```python
from build123d import *

# Parameters (mm, degrees)
SKETCH_1_R          = 2.1
SKETCH_1_R_2        = 1.599999998
SKETCH_1_R_3        = 2.099999998
SKETCH_1_R_4        = 1.6
EXTRUDE_1_DEPTH     = 3
FILLET_1_R          = 2
CUT_EXTRUDE_1_DEPTH = 115.739923305
SKETCH_3_W          = 8.5
SKETCH_3_H          = 7
CUT_EXTRUDE_2_DEPTH = 115.739923305
FILLET_2_R          = 3


with BuildPart() as part:
    # 草图1 → 凸台-拉伸1 (new body)
    with BuildSketch(Plane.XY):
        Polygon((-26, 0), (-26, -62), (26, -62), (26, -51), (96.5, -51), (96.5, -11), (26, -11), (26, 0), align=None)
        with Locations((-20, -4)):
            Circle(SKETCH_1_R, mode=Mode.SUBTRACT)
        with Locations((20, -4)):
            Circle(SKETCH_1_R, mode=Mode.SUBTRACT)
        with Locations((-20, -58)):
            Circle(SKETCH_1_R, mode=Mode.SUBTRACT)
        with Locations((20, -58)):
            Circle(SKETCH_1_R, mode=Mode.SUBTRACT)
        with Locations((42.500000002, -21.5)):
            Circle(SKETCH_1_R_2, mode=Mode.SUBTRACT)
        with Locations((42.500000002, -40.5)):
            Circle(SKETCH_1_R_2, mode=Mode.SUBTRACT)
        with Locations((92.500000002, -18)):
            Circle(SKETCH_1_R_3, mode=Mode.SUBTRACT)
        with Locations((92.500000002, -44)):
            Circle(SKETCH_1_R_3, mode=Mode.SUBTRACT)
        with Locations((25.75, -46)):
            Circle(SKETCH_1_R_4, mode=Mode.SUBTRACT)
        with Locations((25.75, -16)):
            Circle(SKETCH_1_R_4, mode=Mode.SUBTRACT)
        Polygon((68, -34.5), (68, -27.5), (40, -27.5), (40, -19), (24, -19), (24, -43), (40, -43), (40, -34.5), align=None, mode=Mode.SUBTRACT)
    extrude(amount=EXTRUDE_1_DEPTH)

    # 圆角1
    fillet_1_edges = [part.edges().sort_by_distance(p)[0] for p in [
        (26, 0, 1.5),
        (26, -11, 1.5),
        (96.5, -11, 1.5),
        (96.5, -51, 1.5),
        (26, -51, 1.5),
        (26, -62, 1.5),
        (-26, -62, 1.5),
        (-26, 0, 1.5),
        (40, -43, 1.5),
        (40, -34.5, 1.5),
        (68, -34.5, 1.5),
        (68, -27.5, 1.5),
        (40, -27.5, 1.5),
        (40, -19, 1.5),
        (24, -19, 1.5),
        (24, -43, 1.5),
    ]]
    fillet(fillet_1_edges, radius=FILLET_1_R)

    # 草图2 → 切除-拉伸1 (cut, through all)
    with BuildSketch(Plane.XY.offset(3)):
        with BuildLine():
            Line((-18, -28.5), (16, -28.5))
            ThreePointArc((16, -28.5), (18.5, -31), (16, -33.5))
            Line((16, -33.5), (-18, -33.5))
            ThreePointArc((-18, -33.5), (-20.5, -31), (-18, -28.5))
        make_face()
        with BuildLine():
            Line((-18, -20.5), (16, -20.5))
            ThreePointArc((16, -20.5), (18.5, -23), (16, -25.5))
            Line((16, -25.5), (-18, -25.5))
            ThreePointArc((-18, -25.5), (-20.5, -23), (-18, -20.5))
        make_face()
        with BuildLine():
            Line((-18, -12.5), (16, -12.5))
            ThreePointArc((16, -12.5), (18.5, -15), (16, -17.5))
            Line((16, -17.5), (-18, -17.5))
            ThreePointArc((-18, -17.5), (-20.5, -15), (-18, -12.5))
        make_face()
        with BuildLine():
            Line((-18, -36.5), (16, -36.5))
            ThreePointArc((16, -36.5), (18.5, -39), (16, -41.5))
            Line((16, -41.5), (-18, -41.5))
            ThreePointArc((-18, -41.5), (-20.5, -39), (-18, -36.5))
        make_face()
        with BuildLine():
            Line((-18, -44.5), (16, -44.5))
            ThreePointArc((16, -44.5), (18.5, -47), (16, -49.5))
            Line((16, -49.5), (-18, -49.5))
            ThreePointArc((-18, -49.5), (-20.5, -47), (-18, -44.5))
        make_face()
        with BuildLine():
            Line((74.5, -22), (74.5, -40))
            ThreePointArc((74.5, -40), (75.085786438, -41.414213562), (76.5, -42))
            Line((76.5, -42), (84.5, -42))
            ThreePointArc((84.5, -42), (85.914213562, -41.414213562), (86.5, -40))
            Line((86.5, -40), (86.5, -22))
            ThreePointArc((86.5, -22), (85.914213562, -20.585786438), (84.5, -20))
            Line((84.5, -20), (76.5, -20))
            ThreePointArc((76.5, -20), (75.085786438, -20.585786438), (74.5, -22))
        make_face()
    extrude(amount=-CUT_EXTRUDE_1_DEPTH, mode=Mode.SUBTRACT)

    # 草图3 → 切除-拉伸2 (cut, through all)
    with BuildSketch(Plane.XY.offset(3)):
        with Locations((70.25, -31)):
            Rectangle(SKETCH_3_W, SKETCH_3_H)
    extrude(amount=-CUT_EXTRUDE_2_DEPTH, mode=Mode.SUBTRACT)

    # 圆角2
    fillet_2_edges = [part.edges().sort_by_distance(p)[0] for p in [
        (74.5, -27.5, 1.5),
        (74.5, -34.5, 1.5),
    ]]
    fillet(fillet_2_edges, radius=FILLET_2_R)


solid = part.part
```
Check sheet for the modelled part. Datum: model origin and axes. Units: mm. A direction names the side the tool comes from. Coordinates: 2 decimals unless noted, no trailing zeros. Write each loop counter-clockwise with the first axis right and the second up, starting at its lowest first coordinate (ties: lowest second). Pieces come first, ordered by that corner, then holes. Notation, with made-up numbers: M 23,60.5 L 82,60.5 A28 ccw 82,97.5 Z; hole C 75,-12 d5. An arc over 180 degrees is marked long. Write item = value, one per line. Start each with the question number.
1. Thickness scan on probe 1 along Y at (x, z) = (92.5, 1.7); probe 2 along Y at (x, z) = (20, 2.45); probe 3 along Y at (x, z) = (42.5, 0.7). Record the ranges inside material, lowest first.
2. Sectioned sample at B-B (x = 3). Record the cut outline in (y, z), then the cut area to 3 significant figures.
3. Mould release check, pull along Y, two halves, no side actions. Record for faces 3 (the flat face through (-26, -31, 1)), 4 (the flat face through (0, 0, 1)), 5 (the cylindrical face through (18.5, -38.9, 1.5)): pulls with the +Y half, pulls with the -Y half, needs draft (parallel to the pull), parting line crosses it, or undercut.
4. Sectioned sample at D-D (z = 2.4). State how many separate pieces and enclosed holes the cut face has, then the cut area to 3 significant figures.
5. Go/stop test with flat-tipped pins: pin 1 (4 mm diameter, centred on x = -20, y = -4, fed in from +Z); pin 2 (0.9 mm diameter, centred on x = 81, z = 1.5, fed in from +Y). Record where each tip stops, or that it passes through.
6. Tool access check on faces 1 (the flat face through (62, -11, 1)), 2 (the cylindrical face through (-20.5, -39.1, 1.5)). Record the directions out of +Z, -Z, +X, -X, +Y, -Y that give a thin tool (end or side, any length) a straight path to the whole face; none if there is none.
7. Sectioned sample at C-C (x = 92.5). Record the cut outline in (y, z), then the cut area to 3 significant figures.
8. Sectioned sample at A-A (y = -58). Record the cut outline in (x, z), then the cut area to 3 significant figures.
The answers:
q1.probe_1 = -51 to -46.1, -41.9 to -20.1, -15.9 to -11
q1.probe_2 = -62 to -60.1, -55.9 to -6.1, -1.9 to 0
q1.probe_3 = -51 to -42.1, -38.9 to -34.5, -27.5 to -23.1, -19.9 to -11
q2.outline = M -62,0 L -49.5,0 L -49.5,3 L -62,3 Z; M -44.5,0 L -41.5,0 L -41.5,3 L -44.5,3 Z; M -36.5,0 L -33.5,0 L -33.5,3 L -36.5,3 Z; M -28.5,0 L -25.5,0 L -25.5,3 L -28.5,3 Z; M -20.5,0 L -17.5,0 L -17.5,3 L -20.5,3 Z; M -12.5,0 L 0,0 L 0,3 L -12.5,3 Z
q2.area = 111 mm²
q3.face_3 = needs draft
q3.face_4 = pulls with the +Y half
q3.face_5 = undercut
q4.separate_pieces = 1
q4.enclosed_holes = 16
q4.area = 4,090 mm²
q5.pin_1 = through
q5.pin_2 = -11
q6.face_1 = +Z, -Z, +X, +Y
q6.face_2 = +Z, -Z
q7.outline = M -51,0 L -46.1,0 L -46.1,3 L -51,3 Z; M -41.9,0 L -20.1,0 L -20.1,3 L -41.9,3 Z; M -15.9,0 L -11,0 L -11,3 L -15.9,3 Z
q7.area = 94.8 mm²
q8.outline = M -26,0 L -22.1,0 L -22.1,3 L -26,3 Z; M -17.9,0 L 17.9,0 L 17.9,3 L -17.9,3 Z; M 22.1,0 L 26,0 L 26,3 L 22.1,3 Z
q8.area = 131 mm²
